Can you work these out from the drawing? Everything is in mm from the part's minimum corner. A direction names the side the tool comes from. Round coordinates to 2 decimals unless told otherwise and drop trailing zeros. Write each loop counter-clockwise with the first axis right and the second up, starting at its lowest first coordinate (ties: lowest second). Pieces come first, ordered by that corner, then holes. Notation, with made-up numbers: M 86,26.25 L 113,26.25 A15 cw 113,49.25 Z; hole C -14.5,-19.5 d11. An arc over 180 degrees is marked long. Use a Markdown table: item, result. Add a question column.
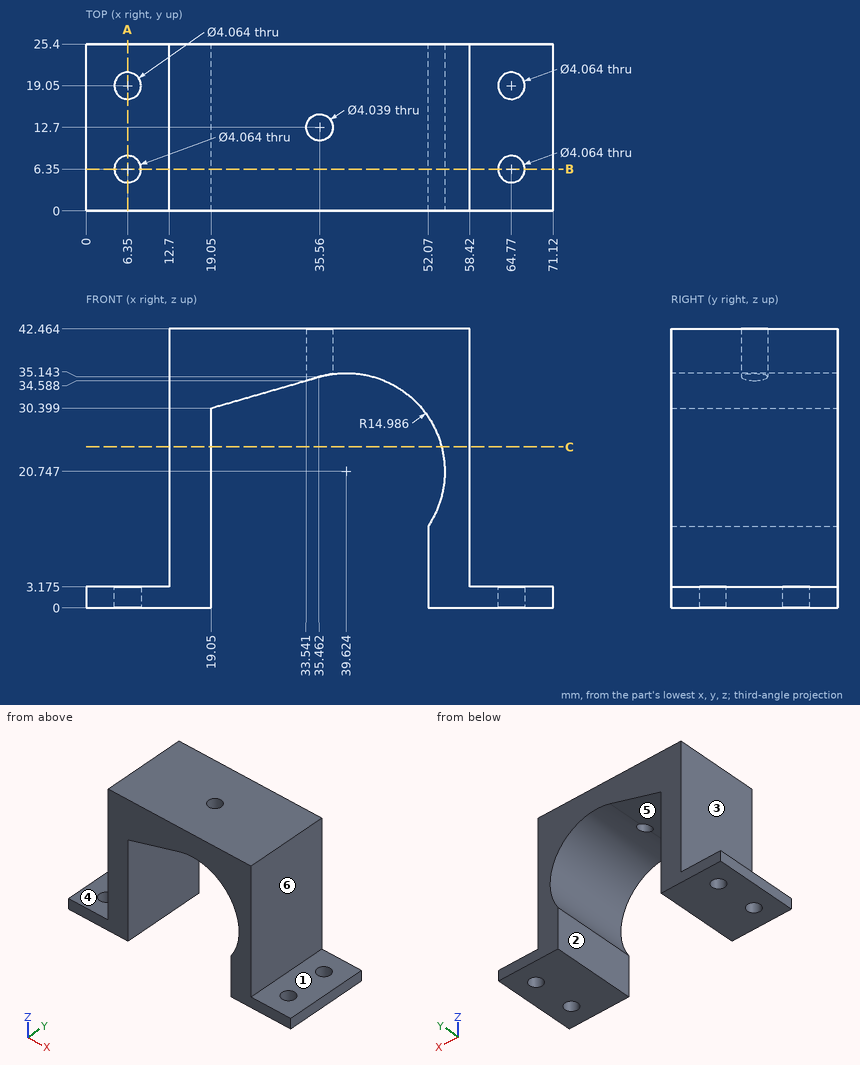
Item 1: On a 3-axis mill with a long thin cutter (end or side, diameter ignored), from which of +Z, -Z, +X, -X, +Y, -Y can I reach the whole of each face in a straight line? I mean the marked faces 1, 2 and 3. Say none if no direction works.
Item 2: Imagine slicing it at A-A on x = 6.35. List the corners of the cut face in (y, z) for me (1 decimal).
Item 3: Imagine slicing it at B-B on y = 6.35. Count the separate pieces of the cut face and the enclosed holes in it.
Item 4: Imagine slicing it at C-C on z = 24.5. List the corners of the cut face in (x, y) for me.
Item 5: For pin 1 Ø6.5 at (x, y) = (64.77, 19.05) entering from +Z (3 decimals); pin 2 Ø7.5 at (y, z) = (14, 16.5) entering from +X; pin 3 Ø2.5 at (x, y) = (35.56, 12.7) entering from +Z; pin 4 Ø3 at (x, y) = (59.5, 21.5) entering from -Z, each with a flat end and sliding along its axis, tell me the tip position at first contact or that it passes through.
Item 6: I need wall thicknesses on probe 1 along Y at (x, z) = (6.35, 0.75); probe 2 along X at (y, z) = (13, 8.5); probe 3 along X at (y, z) = (12, 3). Which ranges of each line are inside material? Lowest first, please. Write a range as from..to.
Item 7: If we mould it in two halves opening along X, with no side actions, what happens to the marked faces 4, 5 and 6? For each: +X half, -X half, draft (parallel to the pull), parting line (faces both ways), or undercut.
The answers:
| question | item | result |
|---|---|---|
| 1 | face 1 | +Z, +X, +Y, -Y |
| 1 | face 2 | -Z, +Y, -Y |
| 1 | face 3 | +Z, -X, +Y, -Y |
| 2 | outline | M 0,0 L 4.3,0 L 4.3,3.2 L 0,3.2 Z; M 8.4,0 L 17,0 L 17,3.2 L 8.4,3.2 Z; M 21.1,0 L 25.4,0 L 25.4,3.2 L 21.1,3.2 Z |
| 3 | separate pieces | 3 |
| 3 | enclosed holes | 0 |
| 4 | outline | M 12.7,0 L 19.05,0 L 19.05,25.4 L 12.7,25.4 Z; M 54.13,0 L 58.42,0 L 58.42,25.4 L 54.13,25.4 Z |
| 5 | pin 1 | z = 3.175 |
| 5 | pin 2 | x = 58.42 |
| 5 | pin 3 | through |
| 5 | pin 4 | z = 0 |
| 6 | probe 1 | 0..4.32, 8.38..17.02, 21.08..25.4 |
| 6 | probe 2 | 12.7..19.05, 52.07..58.42 |
| 6 | probe 3 | 0..19.05, 52.07..71.12 |
| 7 | face 4 | draft |
| 7 | face 5 | undercut |
| 7 | face 6 | +X half |
